Can you work these out from the model? Positions are in its coordinate system, mm. Round coordinates to 2 decimals unless told otherwise and drop trailing zeros. Write each loop counter-clockwise with the first axis right and the second up, starting at its lowest first coordinate (ties: lowest second). Pieces come first, ordered by that corner, then holes.
Q1. If we section it at B-B (y = 70): Please give me the cut outline in (x, z).
Q2. If we section it at A-A (x = 150): Please give me the cut outline in (y, z).
Q3. I'm going to push flat-ended pins straight in: pin 1 Ø2.5 at (x, y) = (120, 90) entering from -Z; pin 2 Ø3.5 at (x, y) = (40, 30) entering from +Z. Where does each tip first touch, or does it pass through?
Q4. Please list where these lines run through material, in increasing order: line 1 along Y through (x, z) = (40, 2.4); line 2 along X through (y, z) = (89, 4.6); line 3 along X through (y, z) = (30, 3.1).
Q5. If we section it at C-C (z = 1.6): Please give me the cut outline in (x, y).
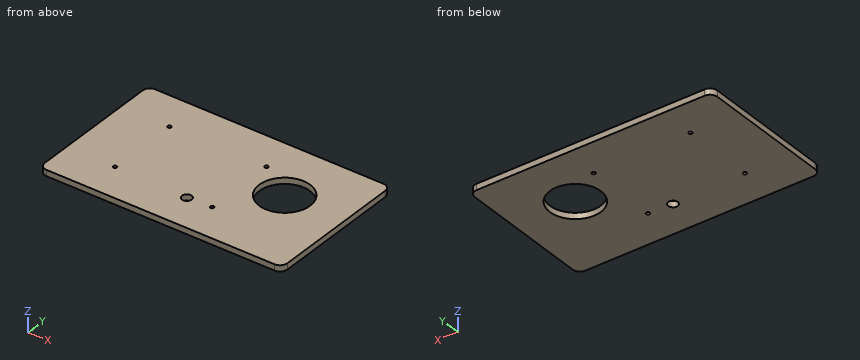
Autodesk Inventor part; units mm, degrees
ref_plane "YZ Plane" through (0, 0, 0) normal (1, 0, 0) x (0, 1, 0)
ref_plane "XZ Plane" through (0, 0, 0) normal (0, 1, 0) x (-1, 0, 0)
ref_plane "XY Plane" through (0, 0, 0) normal (0, 0, 1) x (1, 0, 0)
sketch "Sketch1" plane through (0, 0, 0) normal (0, 0, 1) x (1, 0, 0)
  line L0 (0, 0) -> (200, 0)
  line L1 (200, 0) -> (200, 120)
  line L2 (200, 120) -> (0, 120)
  line L3 (0, 120) -> (0, 0)
  dimension "width" = 200
  dimension "height" = 120
extrude "Extrusion1" add sketch "Sketch1" along normal blind 5
sketch "Sketch2" plane through (0, 0, 5) normal (0, 0, 1) x (1, 0, 0)
  circle A0 centre (150, 70) radius 37
  line L0 (85, 44) -> (115, 44)
  line L1 (115, 44) -> (115, 14)
  line L2 (115, 14) -> (85, 14)
  line L3 (85, 14) -> (85, 44)
  line L4 (0, 120) -> (0, 0)
  line L5 (0, 0) -> (200, 0)
  circle A1 centre (100, 29) radius 4
  circle A2 centre (150, 70) radius 21
  dimension "d4" = 74
  dimension "d5" = 30
  dimension "d6" = 30
  dimension "d7" = 85
  dimension "d8" = 70
  dimension "d9" = 150
  dimension "d10" = 8
  dimension "d11" = 42
extrude "Extrusion2" cut sketch "Sketch2" against normal blind 8 contours A1 | A2
hole "Hole1" at (40, 90, 5) direction (0, 0, -1) diameter 3 end through all
pattern_linear "Rectangular Pattern1" count 2 spacing 80 along (1, 0, 0) count 2 spacing 60 along (0, -1, 0) of "Hole1"
fillet "Fillet1" radius 6 4 edges at (0, 120, 2.5) (0, 0, 2.5) (200, 0, 2.5) (200, 120, 2.5)
properties part number "capac 2"
A:
1. outline: (0, 0) - (129, 0) - (129, 5) - (0, 5) - close; (171, 0) - (200, 0) - (200, 5) - (171, 5) - close
2. outline: (0, 0) - (49, 0) - (49, 5) - (0, 5) - close; (91, 0) - (120, 0) - (120, 5) - (91, 5) - close
3. pin 1: passes through
3. pin 2: stops at z = 5
4. line 1: y = 0 to 28.5, 31.5 to 88.5, 91.5 to 120
4. line 2: x = 0 to 38.88, 41.12 to 118.88, 121.12 to 141.06, 158.94 to 200
4. line 3: x = 0 to 38.5, 41.5 to 96.13, 103.87 to 118.5, 121.5 to 200
5. outline: (0, 6) arc R6 ccw to (6, 0) - (194, 0) arc R6 ccw to (200, 6) - (200, 114) arc R6 ccw to (194, 120) - (6, 120) arc R6 ccw to (0, 114) - close; hole circle Ø3 at (40, 30); hole circle Ø3 at (40, 90); hole circle Ø8 at (100, 29); hole circle Ø3 at (120, 30); hole circle Ø3 at (120, 90); hole circle Ø42 at (150, 70)
